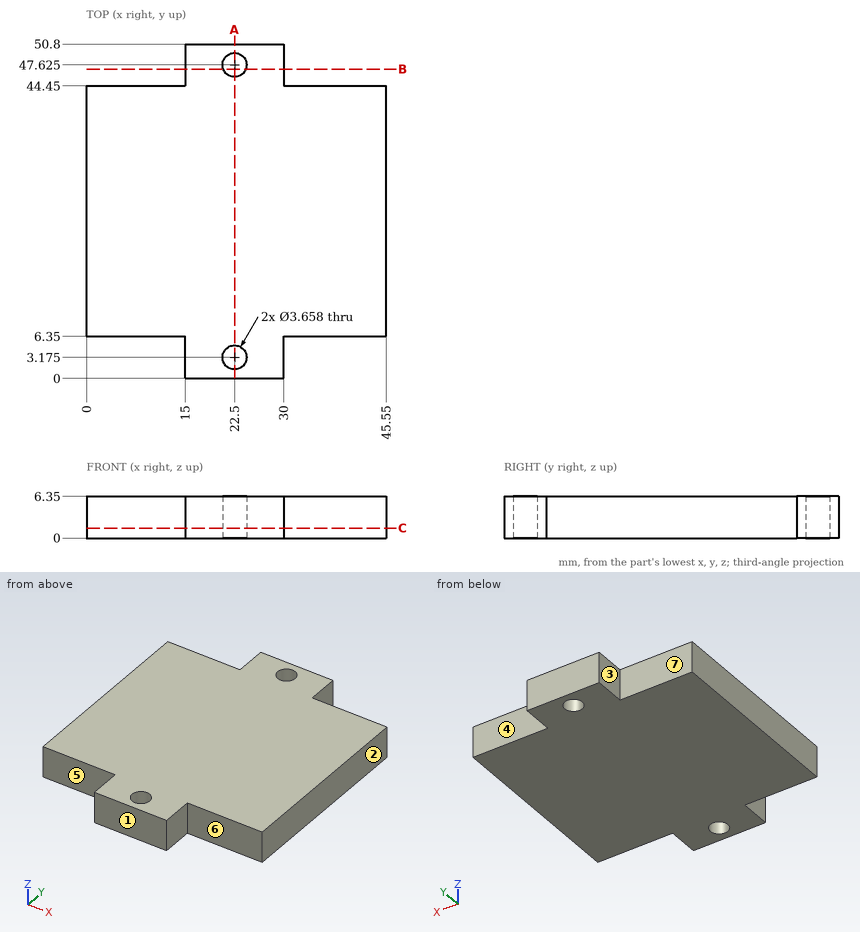
Study the drawing (mm; zero at the part's minimum x, y, z) and answer. A direction names the side the tool comes from. Give positions to 0.01 mm unless a question says otherwise; leave off trailing zeros. Order: outer loops, then holes, each group sorted by start corner. A loop starts at its lowest first (then second) coordinate and runs counter-clockwise, first axis right, second up.
1. Section B-B, the plane y = 47 is taken. Determine the outline of the cut face in (x, z).
Result sheet:
outline: (15, 0) - (20.78, 0) - (20.78, 6.35) - (15, 6.35) - close; (24.22, 0) - (30, 0) - (30, 6.35) - (24.22, 6.35) - close
2. Section A-A, the plane x = 22.5 is taken. Determine the outline of the cut face in (y, z), and give its area (3 significant figures).
Result sheet:
outline: (0, 0) - (1.35, 0) - (1.35, 6.35) - (0, 6.35) - close; (5, 0) - (45.8, 0) - (45.8, 6.35) - (5, 6.35) - close; (49.45, 0) - (50.8, 0) - (50.8, 6.35) - (49.45, 6.35) - close
area: 276 mm2
3. Section C-C, the plane z = 1.5 is taken. Give the number of separate pieces and of enclosed holes in the cut face, and give its area (4 significant figures).
Result sheet:
separate pieces: 1
enclosed holes: 2
area: 1,905 mm2
4. For the marked faces 4, 5, 6 and 7, determine the directions among +Z, -Z, +X, -X, +Y, -Y from which every point of the face is accessible in a straight line to the end or side of a thin tool.
Result sheet:
face 4: +Z, -Z, +X, +Y
face 5: +Z, -Z, -X, -Y
face 6: +Z, -Z, +X, -Y
face 7: +Z, -Z, -X, +Y
5. Straight lines are drawn through the part: L1, parallel to Y at x = 22.5, z = 5.25; L2, parallel to Y at x = 21, z = 5.25; L3, parallel to Y at x = 38, z = 5. For each, find the intervals that lie inside material, in ascending order.
Result sheet:
L1: y = 0 to 1.35, 5 to 45.8, 49.45 to 50.8
L2: y = 0 to 2.13, 4.22 to 46.58, 48.67 to 50.8
L3: y = 6.35 to 44.45
6. Each of these flat-tipped pins is pushed along its axis until it touches: P1, Ø1.9, axis at y = 47, z = 4.5, coming from the -X side; P2, Ø2, axis at x = 22.5, y = 47.625, coming from the +Z side; P3, Ø1.9, axis at x = 5.5, z = 2, coming from the -Y side; P4, Ø6, axis at x = 22.5, y = 3.175, coming from the -Z side. Where does it stop, or does it pass through?
Result sheet:
P1: stops at x = 15
P2: passes through
P3: stops at y = 6.35
P4: stops at z = 0
7. The mould has two halves that part along X. Classify the marked faces 1, 2 and 3: released by +X, released by -X, zero draft, split by the parting line, or undercut.
Result sheet:
face 1: zero draft
face 2: released by +X
face 3: released by -X
